Source: CAD feature listing. Evaluate the final solid. Frame: model axes, mm. Coordinates: 2 decimals unless noted, no trailing zeros. Order: outer loops, then holes, each group sorted by start corner. A loop starts at its lowest first (then second) coordinate and runs counter-clockwise, first axis right, second up.
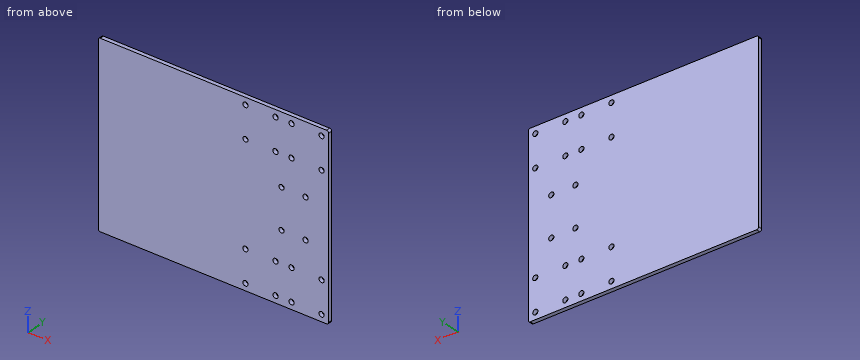
```python
from build123d import *

# Parameters (mm, degrees)
SKETCH_1_W              = 230
SKETCH_1_H              = 180
EXTRUDE_1_DEPTH         = 4
HOLE_WIZARD_5_2_5_2_1_D = 5.2
FILLET_1_R              = 2


with BuildPart() as part:
    # Эскиз1 → Бобышка-Вытянуть1 (new body)
    with BuildSketch(Plane(origin=(0, 0, 0), x_dir=(1, 0, 0), z_dir=(0, 1, 0))):
        with Locations((115, 90)):
            Rectangle(SKETCH_1_W, SKETCH_1_H)
    extrude(amount=EXTRUDE_1_DEPTH)

    # Диаметр отверстия Ø5.2 (5.2)1 (through all)
    with Locations(Plane(origin=(0, 4, 0), x_dir=(1, 0, 0), z_dir=(0, 1, 0))):
        with Locations((183, 70), (183, 110), (207, 70), (207, 110), (223, 39), (223, 7), (193, 7), (193, 39), (147, 39), (177, 39), (147, 7), (177, 7), (193, 173), (223, 173), (223, 141), (193, 141), (177, 173), (147, 173), (177, 141), (147, 141)):
            Hole(HOLE_WIZARD_5_2_5_2_1_D / 2)

    # Скругление1
    fillet_1_edges = [part.edges().sort_by_distance(p)[0] for p in [
        (0, 2, -180),
        (230, 2, -180),
        (230, 2, 0),
        (0, 2, 0),
    ]]
    fillet(fillet_1_edges, radius=FILLET_1_R)


solid = part.part
```
Q1. Pin query (flat end, axial travel): P1, Ø6, axis at x = 183, z = -110, coming from the -Y side. Return the tip coordinate at first contact, or that it passes through.
Solutions:
P1: stops at y = 0
Q2. Section query B-B on z = -70. Output: boundary loops of the cut face in (x, y).
Solutions:
outline: (0, 0) - (180.4, 0) - (180.4, 4) - (0, 4) - close; (185.6, 0) - (204.4, 0) - (204.4, 4) - (185.6, 4) - close; (209.6, 0) - (230, 0) - (230, 4) - (209.6, 4) - close
Q3. Section query C-C on z = -173. Output: boundary loops of the cut face in (x, y).
Solutions:
outline: (0, 0) - (144.4, 0) - (144.4, 4) - (0, 4) - close; (149.6, 0) - (174.4, 0) - (174.4, 4) - (149.6, 4) - close; (179.6, 0) - (190.4, 0) - (190.4, 4) - (179.6, 4) - close; (195.6, 0) - (220.4, 0) - (220.4, 4) - (195.6, 4) - close; (225.6, 0) - (230, 0) - (230, 4) - (225.6, 4) - close
Q4. Section query A-A on x = 177. Output: boundary loops of the cut face in (y, z).
Solutions:
outline: (0, -180) - (4, -180) - (4, -175.6) - (0, -175.6) - close; (0, -170.4) - (4, -170.4) - (4, -143.6) - (0, -143.6) - close; (0, -138.4) - (4, -138.4) - (4, -41.6) - (0, -41.6) - close; (0, -36.4) - (4, -36.4) - (4, -9.6) - (0, -9.6) - close; (0, -4.4) - (4, -4.4) - (4, 0) - (0, 0) - close
Q5. Material intervals for line 1 along Z through (x, y) = (147, 3.1); line 2 along X through (y, z) = (3.05, -141); line 3 along Z through (x, y) = (207, 2.4), sorted ascending.
Solutions:
line 1: z = -180 to -175.6, -170.4 to -143.6, -138.4 to -41.6, -36.4 to -9.6, -4.4 to 0
line 2: x = 0 to 144.4, 149.6 to 174.4, 179.6 to 190.4, 195.6 to 220.4, 225.6 to 230
line 3: z = -180 to -112.6, -107.4 to -72.6, -67.4 to 0
